from build123d import *

# Parameters (mm, degrees)
CYLINDER070_R               = 80
CYLINDER070_DEPTH           = 10
CYLINDER069_R               = 80
CYLINDER069_DEPTH           = 10
BOX005_W                    = 40
BOX005_H                    = 27
BOX005_DEPTH                = 7
BOX004_W                    = 40
BOX004_H                    = 27
BOX004_DEPTH                = 7
CYLINDER071_R               = 12
CYLINDER071_DEPTH           = 10
CYLINDER071_PLACEMENT_ANGLE = 350
BOX002_W                    = 1.75
BOX002_H                    = 27
BOX002_DEPTH                = 7
CYLINDER073_R               = 17.25
CYLINDER073_DEPTH           = 7
CYLINDER067_R               = 17.25
CYLINDER067_DEPTH           = 7
BOX006_W                    = 34.5
BOX006_H                    = 27
BOX006_DEPTH                = 7
CYLINDER072_R               = 19
CYLINDER072_DEPTH           = 7
CYLINDER066_R               = 19
CYLINDER066_DEPTH           = 7
BOX003_W                    = 1.75
BOX003_H                    = 27
BOX003_DEPTH                = 7
CYLINDER076_R               = 12
CYLINDER076_DEPTH           = 10
CYLINDER076_PLACEMENT_ANGLE = 10
CYLINDER077_R               = 7.5
CYLINDER077_DEPTH           = 1.75
CYLINDER075_R               = 7.5
CYLINDER075_DEPTH           = 1.75


with BuildPart() as obj1:
    # Cylinder070 → Cylinder070 (new body)
    with BuildSketch(Plane.XY.offset(-10)):
        Circle(CYLINDER070_R)
    extrude(amount=CYLINDER070_DEPTH)


with BuildPart() as obj2:
    # Cylinder069 → Cylinder069 (new body)
    with BuildSketch(Plane.XY.offset(7)):
        Circle(CYLINDER069_R)
    extrude(amount=CYLINDER069_DEPTH)


with BuildPart() as cube003:
    # Box005 → Box005 (new body)
    with BuildSketch(Plane(origin=(-59, -13.5, 0), x_dir=(1, 0, 0), z_dir=(0, 0, 1))):
        with Locations((20, 13.5)):
            Rectangle(BOX005_W, BOX005_H)
    extrude(amount=BOX005_DEPTH)


with BuildPart() as obj3:
    # Box004 → Box004 (new body)
    with BuildSketch(Plane(origin=(19, -13.5, 0), x_dir=(1, 0, 0), z_dir=(0, 0, 1))):
        with Locations((20, 13.5)):
            Rectangle(BOX004_W, BOX004_H)
    extrude(amount=BOX004_DEPTH)

    # Fusion075: union Cube003
    add(cube003.part)

    # Fusion077: union obj1, obj2
    add(obj1.part)
    add(obj2.part)


with BuildPart() as obj4:
    # Cylinder071 → Cylinder071 (new body)
    with BuildSketch(Plane.XY):
        Circle(CYLINDER071_R)
    extrude(amount=CYLINDER071_DEPTH)


with BuildPart() as obj4_1:
    # Cylinder071 placement: moved
    add(obj4.part.moved(Location((-27.54617, 0, -3.88689))).rotate(Axis((-27.54617, 0, -3.88689), (0, 1, 0)), CYLINDER071_PLACEMENT_ANGLE))


with BuildPart() as obj5:
    # Part__Mirroring: instance of obj4
    add(obj4_1.part.mirror(Plane(origin=(0, 0, 0), x_dir=(0, -1, 0), z_dir=(1, 0, 0))))


with BuildPart() as obj6:
    # Box002 → Box002 (new body)
    with BuildSketch(Plane(origin=(17.25, -13.5, 0), x_dir=(1, 0, 0), z_dir=(0, 0, 1))):
        with Locations((0.875, 13.5)):
            Rectangle(BOX002_W, BOX002_H)
    extrude(amount=BOX002_DEPTH)


with BuildPart() as obj7:
    # Cylinder073 → Cylinder073 (new body)
    with BuildSketch(Plane(origin=(0, -13.5, 0), x_dir=(1, 0, 0), z_dir=(0, 0, 1))):
        Circle(CYLINDER073_R)
    extrude(amount=CYLINDER073_DEPTH)


with BuildPart() as obj8:
    # Cylinder067 → Cylinder067 (new body)
    with BuildSketch(Plane(origin=(0, 13.5, 0), x_dir=(1, 0, 0), z_dir=(0, 0, 1))):
        Circle(CYLINDER067_R)
    extrude(amount=CYLINDER067_DEPTH)


with BuildPart() as obj9:
    # Box006 → Box006 (new body)
    with BuildSketch(Plane(origin=(-17.25, -13.5, 0), x_dir=(1, 0, 0), z_dir=(0, 0, 1))):
        with Locations((17.25, 13.5)):
            Rectangle(BOX006_W, BOX006_H)
    extrude(amount=BOX006_DEPTH)

    # Fusion078: union obj7, obj8
    add(obj7.part)
    add(obj8.part)


with BuildPart() as obj10:
    # Cylinder072 → Cylinder072 (new body)
    with BuildSketch(Plane(origin=(0, -13.5, 0), x_dir=(1, 0, 0), z_dir=(0, 0, 1))):
        Circle(CYLINDER072_R)
    extrude(amount=CYLINDER072_DEPTH)


with BuildPart() as obj11:
    # Cylinder066 → Cylinder066 (new body)
    with BuildSketch(Plane(origin=(0, 13.5, 0), x_dir=(1, 0, 0), z_dir=(0, 0, 1))):
        Circle(CYLINDER066_R)
    extrude(amount=CYLINDER066_DEPTH)

    # Fusion079: union obj10
    add(obj10.part)

    # Cut035: cut obj9
    add(obj9.part, mode=Mode.SUBTRACT)


with BuildPart() as obj12:
    # Box003 → Box003 (new body)
    with BuildSketch(Plane(origin=(-19, -13.5, 0), x_dir=(1, 0, 0), z_dir=(0, 0, 1))):
        with Locations((0.875, 13.5)):
            Rectangle(BOX003_W, BOX003_H)
    extrude(amount=BOX003_DEPTH)


with BuildPart() as obj13:
    # Cylinder076 → Cylinder076 (new body)
    with BuildSketch(Plane.XY):
        Circle(CYLINDER076_R)
    extrude(amount=CYLINDER076_DEPTH)


with BuildPart() as obj13_1:
    # Cylinder076 placement: moved
    add(obj13.part.moved(Location((-27.54617, 0, -3.88689))).rotate(Axis((-27.54617, 0, -3.88689), (0, -1, 0)), CYLINDER076_PLACEMENT_ANGLE))

    # Fusion080: union obj5, obj6, obj11, obj12
    add(obj5.part)
    add(obj6.part)
    add(obj11.part)
    add(obj12.part)

    # Cut036: cut obj3
    add(obj3.part, mode=Mode.SUBTRACT)


with BuildPart() as fingertab1:
    # Cylinder077 → Cylinder077 (new body)
    with BuildSketch(Plane(origin=(0, -30.75, 3.5), x_dir=(1, 0, 0), z_dir=(0, -1, 0))):
        Circle(CYLINDER077_R)
    extrude(amount=CYLINDER077_DEPTH)


with BuildPart() as fingertab:
    # Cylinder075 → Cylinder075 (new body)
    with BuildSketch(Plane(origin=(0, -30.75, 3.5), x_dir=(1, 0, 0), z_dir=(0, -1, 0))):
        Circle(CYLINDER075_R)
    extrude(amount=CYLINDER075_DEPTH)


with BuildPart() as toplevelpart_lockring:
    # Part__Mirroring010: instance of FingerTab
    add(fingertab.part.mirror(Plane(origin=(0, 0, 0), x_dir=(1, 0, 0), z_dir=(0, 1, 0))))

    # Fusion081: union obj13, FingerTab1
    add(obj13_1.part)
    add(fingertab1.part)


solid = toplevelpart_lockring.part
Part model, mm, in its own coordinate system. A direction names the side the tool comes from. Give positions to 0.01 mm unless a question says otherwise; leave off trailing zeros. Write each loop counter-clockwise with the first axis right and the second up, starting at its lowest first coordinate (ties: lowest second). Pieces come first, ordered by that corner, then holes.
1) Two-plate mould, pull along Y, no slides. Class faces 6 (the face through (-15.512, 24.471, 3.451)), 7 (the face through (15.512, -24.471, 3.451)), 8 (the face through (16.506, -0.075, 2.607)): released by +Y, released by -Y, zero draft, split by the parting line, or undercut.
Resolved:
face 6: released by +Y
face 7: released by -Y
face 8: undercut
2) Cut at B-B on y = -11. Write the cut outline in (x, z).
Resolved:
outline: (-19, 0) - (-17.25, 0) - (-17.25, 7) - (-19, 7) - close; (17.25, 0) - (19, 0) - (19, 7) - (17.25, 7) - close
3) Which spindle directions (+Z, -Z, +X, -X, +Y, -Y) get a long thin tool onto all of the face, cutting with end or side? Do faces 1 (the face through (0, 30.75, 9)), 2 (the face through (-7.493, 31.613, 3.83)), 3 (the face through (-16.506, -0.075, 2.607)), 4 (the face through (0.379, 30.746, 3.451)), 5 (the face through (0, 30.75, -2)). Say none if no direction does.
Resolved:
face 1: +Z, +X, -X
face 2: +Y
face 3: +Z
face 4: +Z, -Z
face 5: -Z, +X, -X
4) Pin check, flat tips, straight feed: pin 1 (21 mm diameter, centred on x = -10, y = -13, fed in from -Z); pin 2 (6 mm diameter, centred on x = -10, z = -2, fed in from -Y); pin 3 (1.5 mm diameter, centred on x = 13, z = 6, fed in from -Y). Stop position of each tip, or through.
Resolved:
pin 1: stops at z = 0
pin 2: stops at y = -30.84
pin 3: stops at y = -28.02
5) Probe L1, parallel to Y at x = -5, z = -0.5; L2, parallel to X at y = -12, z = 0.25; L3, parallel to Y at x = 2, z = 4.5. List the from-to ranges inside material, lowest first.
Resolved:
L1: y = -32.5 to -30.75, 30.75 to 32.5
L2: x = -19 to -17.25, 17.25 to 19
L3: y = -32.5 to -30.63, 30.63 to 32.5
6) Cut at A-A on z = 8. Write the cut outline in (x, y).
Resolved:
outline: (-6, -32.5) - (6, -32.5) - (6, -30.75) - (-6, -30.75) - close; (-6, 30.75) - (6, 30.75) - (6, 32.5) - (-6, 32.5) - close
